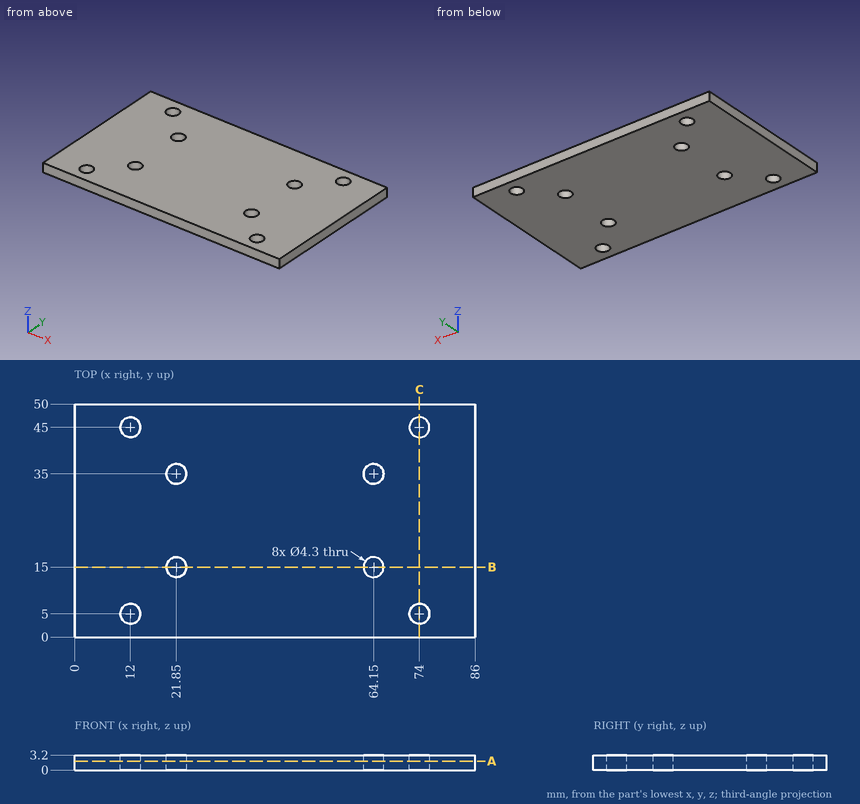
For this review, use the dimensioned drawing (mm, ordinates from the lowest corner) and the shaded views. Give positions to 0.01 mm unless a question says otherwise; leave off trailing zeros. Write each loop counter-clockwise with the first axis right and the second up, starting at its lowest first coordinate (ties: lowest second). Pieces come first, ordered by that corner, then holes. Notation, with made-up numbers: M 33,-20.5 L 68,-20.5 A30 cw 68,18.5 Z; hole C 6.25,-0.75 d7. An arc over 180 degrees is marked long. Answer as a JSON object with one key per item and string values. Group by question number.
1) We need section C-C (x = 74). Give the boundary of the cut face in (y, z).
2) We need section B-B (y = 15). Give the boundary of the cut face in (x, z).
3) We need section A-A (z = 1.9). Count the separate pieces of the cut face and the enclosed holes in it, and give its area (3 significant figures).
4) Clearance check with a flat-ended pin moving along its axis: pin 1 Ø5 at (x, y) = (12, 45) entering from +Z. State where the tip first meets the part, or that it passes through.
5) For line 1 along Y through (x, z) = (64.15, 1.55); line 2 along X through (y, z) = (35, 2.2); line 3 along Y through (x, z) = (12, 1.5), list the stretches that pass through material, from the lowest coordinate up.
Answer key:
{
 "1": {"outline": "M 0,0 L 2.85,0 L 2.85,3.2 L 0,3.2 Z; M 7.15,0 L 42.85,0 L 42.85,3.2 L 7.15,3.2 Z; M 47.15,0 L 50,0 L 50,3.2 L 47.15,3.2 Z"},
 "2": {"outline": "M 0,0 L 19.7,0 L 19.7,3.2 L 0,3.2 Z; M 24,0 L 62,0 L 62,3.2 L 24,3.2 Z; M 66.3,0 L 86,0 L 86,3.2 L 66.3,3.2 Z"},
 "3": {"separate pieces": "1", "enclosed holes": "8", "area": "4,180 mm²"},
 "4": {"pin 1": "stops at z = 3.2"},
 "5": {"line 1": "y = 0 to 12.85, 17.15 to 32.85, 37.15 to 50", "line 2": "x = 0 to 19.7, 24 to 62, 66.3 to 86", "line 3": "y = 0 to 2.85, 7.15 to 42.85, 47.15 to 50"}
}
